The figure shows three views and two pictorial views of one solid part (mm, origin at its lowest corner). Answer the questions. A direction names the side the tool comes from. Give positions to 0.01 mm unless a question says otherwise; leave off trailing zeros. Write each loop counter-clockwise with the first axis right and the second up, starting at its lowest first coordinate (ties: lowest second). Pieces come first, ordered by that corner, then holes. Notation, with made-up numbers: M 61,-23.5 L 65,-23.5 A29 ccw 65,10.5 Z; hole C 0.5,-34 d7. An arc over 180 degrees is marked long. Return JSON: item names as keys, results as strings.
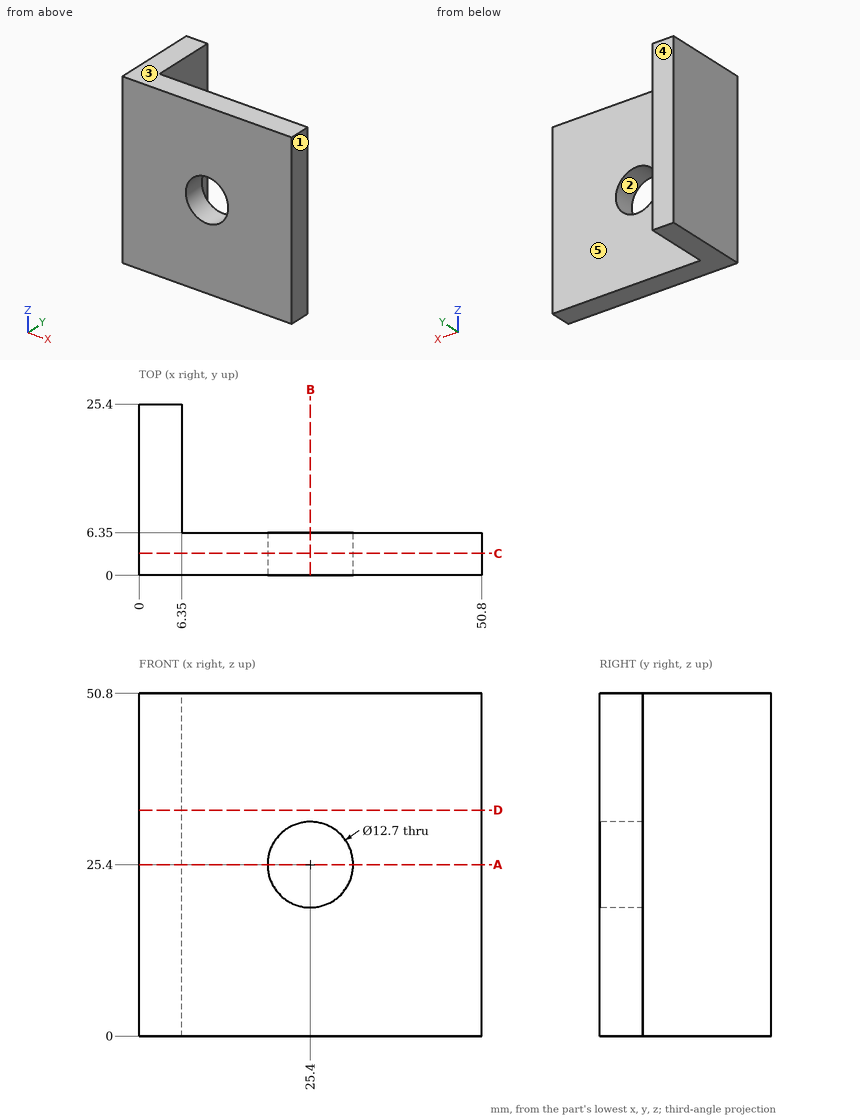
Item 1: Given pin 1 Ø8 at (x, z) = (35, 32.5) entering from +Y; pin 2 Ø15 at (y, z) = (17, 20.5) entering from +X, each flat-ended and moving along its own axis, determine where each tip first touches the part or whether it passes through.
Geometry results:
{"pin 1": "stops at y = 6.35", "pin 2": "stops at x = 6.35"}
Item 2: A cutting plane is placed at D-D, the plane z = 33.5. Write down the section's boundary in (x, y).
Geometry results:
{"outline": "M 0,0 L 50.8,0 L 50.8,6.35 L 6.35,6.35 L 6.35,25.4 L 0,25.4 Z"}
Item 3: A cutting plane is placed at C-C, the plane y = 3.25. Write down the section's boundary in (x, z), plus the area to 3 significant figures.
Geometry results:
{"outline": "M 0,0 L 50.8,0 L 50.8,50.8 L 0,50.8 Z; hole C 25.4,25.4 d12.7", "area": "2,450 mm2"}
Item 4: Determine the mould class of the marked faces 1, 2 and 3 for opening direction Z: +Z half, -Z half, draft (parallel to the pull), parting line (faces both ways), or undercut.
Geometry results:
{"face 1": "draft", "face 2": "undercut", "face 3": "+Z half"}
Item 5: Which of the six approach directions +Z, -Z, +X, -X, +Y, -Y give full straight-line access (tool end or side, diameter ignored) to the marked faces 4 and 5?
Geometry results:
{"face 4": "+Z, -Z, +X, -X, +Y", "face 5": "+Z, -Z, +X, +Y"}
Item 6: Find the intervals of material crossed by line 1 (Z direction, x = 25.4, y = 2); line 2 (Y direction, x = 30, z = 17), in increasing order.
Geometry results:
{"line 1": "z = 0 to 19.05, 31.75 to 50.8", "line 2": "y = 0 to 6.35"}
Item 7: A cutting plane is placed at B-B, the plane x = 25.4. Write down the section's boundary in (y, z), plus the area to 3 significant figures.
Geometry results:
{"outline": "M 0,0 L 6.35,0 L 6.35,19.05 L 0,19.05 Z; M 0,31.75 L 6.35,31.75 L 6.35,50.8 L 0,50.8 Z", "area": "242 mm2"}
Item 8: A cutting plane is placed at A-A, the plane z = 25.4. Write down the section's boundary in (x, y).
Geometry results:
{"outline": "M 0,0 L 19.05,0 L 19.05,6.35 L 6.35,6.35 L 6.35,25.4 L 0,25.4 Z; M 31.75,0 L 50.8,0 L 50.8,6.35 L 31.75,6.35 Z"}
